Can you work these out from the model? Positions are in its coordinate system, mm. A direction names the side the tool comes from. Give positions to 0.01 mm unless a question says otherwise; leave off trailing zeros. Loops run counter-clockwise (first coordinate to the right, second up) from the corner with the lowest first, then second, coordinate; pieces in that order, holes last. Notation, with made-up numbers: (89, 10) -> (110, 10) arc R27 ccw to (110, 31) -> close; hole circle Ø5 at (53.25, -2.75). An arc over 180 degrees is marked (long way). One line per question, with ' | ' between items.
from build123d import *

# Parameters (mm, degrees)
F0_W      = 125
F0_H      = 25
F1_DEPTH  = 55
F2_W      = 5
F2_H      = 30
F3_DEPTH  = 125.001
F4_W      = 125
F4_H      = 10
F5_DEPTH  = 40
F6_R      = 20
F7_R      = 20
F8_SIZE   = 10
F9_SIZE   = 10
F10_R     = 15
F11_DEPTH = 25.001


with BuildPart() as f1:
    # F0 (on Front) → F1 (new body)
    with BuildSketch(Plane.XZ):
        Rectangle(F0_W, F0_H)
    extrude(amount=F1_DEPTH)

    # F2 (on face) → F3 (cut, through all)
    with BuildSketch(Plane(origin=(-62.5, 0, 0), x_dir=(0, -1, 0), z_dir=(-1, 0, 0))):
        with Locations((47.5, -12.5)):
            Rectangle(F2_W, F2_H)
    extrude(amount=-F3_DEPTH, mode=Mode.SUBTRACT)

    # F4 (on face) → F5 (join)
    with BuildSketch(Plane.XY.offset(12.5)):
        with Locations((0, -47.5)):
            Rectangle(F4_W, F4_H)
        with Locations((0, -7.5)):
            Rectangle(F4_W, F4_H)
    extrude(amount=F5_DEPTH)

    # F6
    f6_edges = [f1.edges().sort_by_distance(p)[0] for p in [
        (-62.5, -47.5, 52.5),
    ]]
    fillet(f6_edges, radius=F6_R)

    # F7
    f7_edges = [f1.edges().sort_by_distance(p)[0] for p in [
        (62.5, -7.5, 52.5),
    ]]
    fillet(f7_edges, radius=F7_R)

    # F8
    f8_edges = [f1.edges().sort_by_distance(p)[0] for p in [
        (62.5, -47.5, 52.5),
    ]]
    chamfer(f8_edges, length=F8_SIZE)

    # F9
    f9_edges = [f1.edges().sort_by_distance(p)[0] for p in [
        (-62.5, -7.5, 52.5),
    ]]
    chamfer(f9_edges, length=F9_SIZE)

    # F10 (on face) → F11 (cut, through all)
    with BuildSketch(Plane.XY.offset(12.5)):
        with Locations((0, -27.5)):
            Circle(F10_R)
    extrude(amount=-F11_DEPTH, mode=Mode.SUBTRACT)


solid = f1.part
Q1. If we section it at D-D (x = 31.5): Write out the boundary of the cut face in (y, z), plus the area to 3 significant figures.
Entries:
outline: (-55, -12.5) -> (-50, -12.5) -> (-50, 2.5) -> (-45, 2.5) -> (-45, -12.5) -> (0, -12.5) -> (0, 12.5) -> (-2.5, 12.5) -> (-2.5, 52.5) -> (-12.5, 52.5) -> (-12.5, 12.5) -> (-42.5, 12.5) -> (-42.5, 52.5) -> (-52.5, 52.5) -> (-52.5, 12.5) -> (-55, 12.5) -> close | area: 2,100 mm²
Q2. If we section it at A-A (z = -8.5): Write out the boundary of the cut face in (x, y).
Entries:
outline: (-62.5, -55) -> (62.5, -55) -> (62.5, -50) -> (-62.5, -50) -> close; (-62.5, -45) -> (62.5, -45) -> (62.5, 0) -> (-62.5, 0) -> close; hole circle Ø30 at (0, -27.5)
Q3. For pin 1 Ø10 at (x, y) = (27, -28) entering from +Z; pin 2 Ø12 at (x, z) = (-20.5, 27.5) entering from +Y; pin 3 Ø20 at (x, z) = (-8, 27.5) entering from -Y; pin 4 Ø12 at (x, z) = (-18, -7) entering from +Y, each with a flat end and sliding along its axis, tell me the tip position at first contact or that it passes through.
Entries:
pin 1: z = 12.5 | pin 2: y = -2.5 | pin 3: y = -52.5 | pin 4: y = 0
Q4. If we section it at C-C (z = 15): Write out the boundary of the cut face in (x, y), plus the area to 3 significant figures.
Entries:
outline: (-62.5, -52.5) -> (62.5, -52.5) -> (62.5, -42.5) -> (-62.5, -42.5) -> close; (-62.5, -12.5) -> (62.5, -12.5) -> (62.5, -2.5) -> (-62.5, -2.5) -> close | area: 2,500 mm²
Q5. If I drill on probe 1 along Y at (x, z) = (0, -1.25); probe 2 along Y at (x, z) = (-24, 35); probe 3 along Y at (x, z) = (0, 4), over which ranges is the centre line in solid material (lowest first)? Write a range as from..to.
Entries:
probe 1: -55..-50, -45..-42.5, -12.5..0 | probe 2: -52.5..-42.5, -12.5..-2.5 | probe 3: -55..-42.5, -12.5..0
Q6. On a 3-axis mill with a long thin cutter (end or side, diameter ignored), from which of +Z, -Z, +X, -X, +Y, -Y can I reach the whole of each face in a straight line? I mean faces 1 (the face through (56.486, -7.43, 46.797)), 2 (the face through (-1, -45, -5)), 3 (the face through (-1, -42.5, 32)), 4 (the face through (-1, -1, 12.5)). Say none if no direction works.
Entries:
face 1: +Z, +X, +Y | face 2: -Z, +X, -X | face 3: +Z, +X, -X | face 4: +Z, +X, -X, +Y
Q7. If we section it at B-B (y = -27.5): Write out the boundary of the cut face in (x, z).
Entries:
outline: (-62.5, -12.5) -> (-15, -12.5) -> (-15, 12.5) -> (-62.5, 12.5) -> close; (15, -12.5) -> (62.5, -12.5) -> (62.5, 12.5) -> (15, 12.5) -> close
